from build123d import *

# Parameters (mm, degrees)
SKETCH1_W           = 20
SKETCH1_H           = 105
BOSS_EXTRUDE1_DEPTH = 5
SKETCH2_R           = 3.175
CUT_EXTRUDE1_DEPTH  = 54.677276384
SKETCH4_W           = 20
SKETCH4_H           = 50
BOSS_EXTRUDE3_DEPTH = 19
SKETCH5_R           = 3.5
CUT_EXTRUDE2_DEPTH  = 3
FILLET5_R           = 10


with BuildPart() as part:
    # Sketch1 → Boss-Extrude1 (new body)
    with BuildSketch(Plane.XY):
        Rectangle(SKETCH1_W, SKETCH1_H)
    extrude(amount=BOSS_EXTRUDE1_DEPTH)

    # Sketch2 → Cut-Extrude1 (cut, through all)
    with BuildSketch(Plane.XY.offset(5)):
        with Locations((0, 37.5)):
            Circle(SKETCH2_R)
        with Locations((0, -37.5)):
            Circle(SKETCH2_R)
    extrude(amount=-CUT_EXTRUDE1_DEPTH, mode=Mode.SUBTRACT)

    # Sketch4 → Boss-Extrude3 (add)
    with BuildSketch(Plane.XY.offset(5)):
        Rectangle(SKETCH4_W, SKETCH4_H)
    extrude(amount=BOSS_EXTRUDE3_DEPTH)

    # Sketch5 → Cut-Extrude2 (cut)
    with BuildSketch(Plane.XY.offset(24)):
        with Locations((0, -15)):
            Circle(SKETCH5_R)
        with Locations((0, 15)):
            Circle(SKETCH5_R)
    extrude(amount=-CUT_EXTRUDE2_DEPTH, mode=Mode.SUBTRACT)

    # Fillet5
    fillet5_edges = [part.edges().sort_by_distance(p)[0] for p in [
        (10, -52.5, 2.5),
        (-10, -52.5, 2.5),
        (10, -25, 14.5),
        (-10, -25, 14.5),
        (10, 25, 14.5),
        (-10, 25, 14.5),
        (-10, 52.5, 2.5),
        (10, 52.5, 2.5),
    ]]
    fillet(fillet5_edges, radius=FILLET5_R - 0.0001)  # a hair under: the kernel refuses the full size


solid = part.part
The listing builds one solid part. Answer for the finished solid, in the listing's coordinates (mm). A direction names the side the tool comes from. Give positions to 0.01 mm unless a question says otherwise; leave off trailing zeros. Write each loop counter-clockwise with the first axis right and the second up, starting at its lowest first coordinate (ties: lowest second). Pieces come first, ordered by that corner, then holes. Notation, with made-up numbers: (45.5, -16) -> (74.5, -16) arc R15 cw to (74.5, 13) -> close; hole circle Ø4 at (45.5, 86.25). An arc over 180 degrees is marked (long way). One line per question, with ' | ' between items. Start each with the question number.
1. Section C-C (x = -2) is taken. Determine the outline of the cut face in (y, z).
2. Section B-B (y = -37.5) is taken. Determine the outline of the cut face in (x, z) (3 decimals), plus the area to 4 significant figures.
3. Given pin 1 Ø12 at (x, y) = (-1, 33.5) entering from +Z; pin 2 Ø3 at (x, z) = (4, 5) entering from +Y; pin 3 Ø4 at (x, z) = (-4, 18.5) entering from +Y, each flat-ended and moving along its own axis, determine where each tip first touches the part or whether it passes through.
4. For faces 4 (the cylindrical face through (6.99, 22.15, 14.63)), 5 (the cylindrical face through (-7.15, 21.99, 14.63)), 6 (the flat face through (-10, -1, 9)), 7 (the cylindrical face through (-0.759, 11.583, 22.521)), 8 (the cylindrical face through (6.99, -22.15, 14.63)), determine the directions among +Z, -Z, +X, -X, +Y, -Y from which every point of the face is accessible in a straight line to the end or side of a thin tool.
5. Section A-A (z = 2) is taken. State how many separate pieces and enclosed holes the cut face has, plus the area to 3 significant figures.
6. Find the intervals of material crossed by probe 1 along Y at (x, z) = (0, 3.2) (3 decimals); probe 2 along Y at (x, z) = (0, 22.2); probe 3 along Z at (x, y) = (0.5, -12), in increasing order.
7. For a pull along Y with two mould halves and no side action, classify faces 1 (the cylindrical face through (-0.69, 34.4, 2.54)), 2 (the flat face through (0, 34, 5)), 3 (the cylindrical face through (-7.15, -21.99, 14.63)) as pulls with the +Y half, pulls with the -Y half, needs draft (parallel to the pull), parting line crosses it, or undercut.
Response values:
1) outline: (-52.3, 0) -> (-39.97, 0) -> (-39.97, 5) -> (-52.3, 5) -> close; (-35.03, 0) -> (35.03, 0) -> (35.03, 5) -> (24.8, 5) -> (24.8, 24) -> (17.87, 24) -> (17.87, 21) -> (12.13, 21) -> (12.13, 24) -> (-12.13, 24) -> (-12.13, 21) -> (-17.87, 21) -> (-17.87, 24) -> (-24.8, 24) -> (-24.8, 5) -> (-35.03, 5) -> close; (39.97, 0) -> (52.3, 0) -> (52.3, 5) -> (39.97, 5) -> close
2) outline: (-10, 0) -> (-3.175, 0) -> (-3.175, 5) -> (-10, 5) -> close; (3.175, 0) -> (10, 0) -> (10, 5) -> (3.175, 5) -> close | area: 68.25 mm2
3) pin 1: z = 5 | pin 2: y = 52.18 | pin 3: y = 24.8
4) face 4: +Z, +X, +Y | face 5: +Z, -X, +Y | face 6: +Z, -Z, -X, +Y, -Y | face 7: +Z | face 8: +Z, +X, -Y
5) separate pieces: 1 | enclosed holes: 2 | area: 1,950 mm2
6) probe 1: -52.5 to -40.675, -34.325 to 34.325, 40.675 to 52.5 | probe 2: -25 to -18.5, -11.5 to 11.5, 18.5 to 25 | probe 3: 0 to 21
7) face 1: undercut | face 2: needs draft | face 3: pulls with the -Y half
